```python
from build123d import *

# Parameters (mm, degrees)
F1_DEPTH  = 50
F3_START  = 1
F3_DEPTH  = 48
F4_R      = 2.5
F5_DEPTH  = 3
F6_R      = 4
F7_DEPTH  = 5
F8_R      = 1
F9_DEPTH  = 10
F10_R     = 3.75
F11_DEPTH = 2


with BuildPart() as f1:
    # F0 (on Top) → F1 (new body)
    with BuildSketch(Plane.XY):
        with BuildLine():
            Line((0, 0), (-25, 43.3012701892))
            ThreePointArc((-25, 43.3012701892), (-43.3012701892, 25), (-50, 0))
            Line((-50, 0), (0, 0))
        make_face()
    extrude(amount=F1_DEPTH)

    # F2 (on Top) → F3 (cut)
    with BuildSketch(Plane.XY.offset(F3_START)):
        with BuildLine():
            Line((-1.7320508076, 1), (-25.3609228316, 41.9264068712))
            ThreePointArc((-25.3609228316, 41.9264068712), (-42.4352447854, 24.5), (-48.9897948557, 1))
            Line((-48.9897948557, 1), (-1.7320508076, 1))
        make_face()
    extrude(amount=F3_DEPTH, mode=Mode.SUBTRACT)

    # F4 (on face) → F5 (join)
    with BuildSketch(Plane(origin=(0, 0, 0), x_dir=(1, 0, 0), z_dir=(0, 0, -1))):
        with Locations((-40.7031939779, -23.5)):
            Circle(F4_R)
    extrude(amount=F5_DEPTH)

    # F6 (on face) → F7 (join)
    with BuildSketch(Plane(origin=(0, 0, -3), x_dir=(1, 0, 0), z_dir=(0, 0, -1))):
        with Locations((-40.7031939779, -23.5)):
            Circle(F6_R)
    extrude(amount=F7_DEPTH)

    # F8 (on face) → F9 (join)
    with BuildSketch(Plane(origin=(0, 0, -8), x_dir=(1, 0, 0), z_dir=(0, 0, -1))):
        with Locations((-40.7031939779, -23.5)):
            Circle(F8_R)
    extrude(amount=F9_DEPTH)

    # F10 (on face) → F11 (cut)
    with BuildSketch(Plane.XY.offset(50)):
        with Locations((-34.6410161514, 20)):
            Circle(F10_R)
    extrude(amount=-F11_DEPTH, mode=Mode.SUBTRACT)


solid = f1.part
```
Model file for the job. Use its own axes, mm. A direction names the side the tool comes from. Coordinates: 2 decimals unless noted, no trailing zeros. Loops run counter-clockwise (first coordinate to the right, second up) from the corner with the lowest first, then second, coordinate; pieces in that order, holes last. Notation, with made-up numbers: (0, 11.5) - (27, 11.5) arc R6 ccw to (27, 15.5) - close; hole circle Ø6 at (-24.5, 49). An arc over 180 degrees is marked (long way). Answer as a JSON object with one key per item and string values. Group by question number.
(1) Cut at D-D (z = -2). Give the cut face in (x, y), then the cut area to 3 significant figures.
(2) Cut at A-A (x = -21.5). Give the cut face in (y, z), then the cut area to 3 significant figures.
(3) Cut at C-C (z = 5.5). Give the cut face in (x, y), then the cut area to 3 significant figures.
(4) Cut at B-B (y = 29.5). Give the cut face in (x, z).
(5) Tool access for faces 4 (the face through (-40.92, 24.476, -12.93)), 5 (the face through (-37.62, 17.72, 49.51)), 6 (the face through (-41.03, 21.02, -1.48)): list every direction of +Z, -Z, +X, -X, +Y, -Y with a clear straight run to the whole face (end or side of a thin tool).
(6) Two-plate mould, pull along Z, no slides. Class faces 1 (the face through (-39.87, 24.33, -8)), 2 (the face through (-43, 25, -3)), 3 (the face through (-36.888, 22.299, -5.465)): released by +Z, released by -Z, zero draft, split by the parting line, or undercut.
(7) Flat gauge pins, fed straight in: pin 1 (3 mm diameter, centred on y = 28, z = 39, fed in from +X); pin 2 (3 mm diameter, centred on x = -25.5, z = 30.5, fed in from +Y); pin 3 (6 mm diameter, centred on y = 20, z = 19.5, fed in from -X); pin 4 (10 mm diameter, centred on x = -34.64, y = 20, fed in from -Z). Where does each tip first touch, or does it go through?
(8) Probe line 1 along Z through (x, y) = (-30, 18); line 2 along X through (y, z) = (29, 24); line 3 along Y through (x, z) = (-10.5, 37). List the from-to ranges inside material, lowest first.
Geometry says:
{
 "1": {"outline": "circle Ø5 at (-40.7, 23.5)", "area": "19.6 mm^2"},
 "2": {"outline": "(0, 0) - (37.24, 0) - (37.24, 50) - (0, 50) - close; hole (1, 1) - (35.24, 1) - (35.24, 49) - (1, 49) - close", "area": "218 mm^2"},
 "3": {"outline": "(-50, 0) - (0, 0) - (-25, 43.3) arc R50 ccw to start; hole (-48.99, 1) - (-1.73, 1) - (-25.36, 41.93) arc R49 ccw to start", "area": "148 mm^2"},
 "4": {"outline": "(-40.37, 0) - (-17.03, 0) - (-17.03, 50) - (-40.37, 50) - close; hole (-39.12, 1) - (-18.19, 1) - (-18.19, 49) - (-39.12, 49) - close"},
 "5": {"face 4": "-Z", "face 5": "+Z", "face 6": "none"},
 "6": {"face 1": "released by -Z", "face 2": "undercut", "face 3": "zero draft"},
 "7": {"pin 1": "stops at x = -15.3", "pin 2": "stops at y = 43.3", "pin 3": "stops at x = -47.02", "pin 4": "stops at z = -8"},
 "8": {"line 1": "z = 0 to 1, 49 to 50", "line 2": "x = -40.73 to -39.5, -17.9 to -16.74", "line 3": "y = 0 to 1, 16.19 to 18.19"}
}
